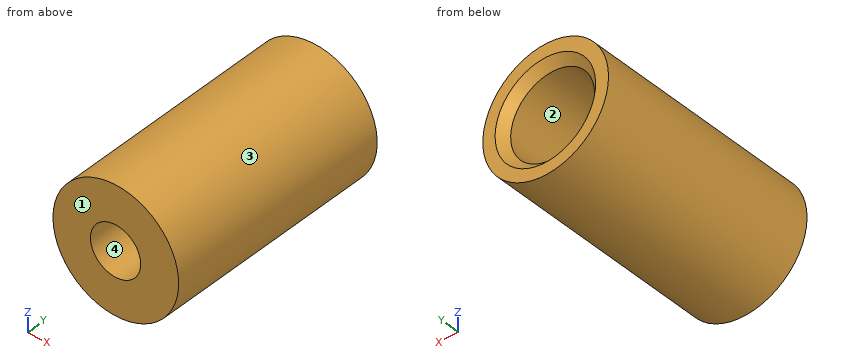
Autodesk Inventor part; units mm, degrees
ref_plane "YZ Plane" through (0, 0, 0) normal (1, 0, 0) x (0, 1, 0)
ref_plane "XZ Plane" through (0, 0, 0) normal (0, 1, 0) x (-1, 0, 0)
ref_plane "XY Plane" through (0, 0, 0) normal (0, 0, 1) x (1, 0, 0)
sketch "Эскиз1" plane through (0, 0, 0) normal (0, 1, 0) x (-1, 0, 0)
  circle A0 centre (0, 0) radius 15
  dimension "d0" = 30
extrude "Выдавливание1" add sketch "Эскиз1" along normal blind 55
hole "Отверстие1" at (-0.0551, 55, -0.1504) direction (0, -1, 0) diameter 12 depth 55 tip angle 118
hole "Отверстие2" at (0.0739, 55, -0.1164) direction (0, -1, 0) diameter 20 depth 25 tip angle 118
thread "Резьба1"
chamfer "Фаска1" distance 2 angle 45 1 edges at (0.0739, 55, -10.1164)
The listing builds one solid part. Answer for the finished solid, in the listing's coordinates (mm). Face numbers are marked on the shaded views. Round coordinates to 2 decimals unless told otherwise and drop trailing zeros. Write each loop counter-clockwise with the first axis right and the second up, starting at its lowest first coordinate (ties: lowest second). Pieces come first, ordered by that corner, then holes. Notation, with made-up numbers: M 47,35.5 L 55,35.5 A28 ccw 55,63.5 Z; hole C 4.25,46 d11. An arc over 180 degrees is marked long. Write each question's results on one line, items separated by ' | '. Start each with the question number.
Item 1: Find section B-B on y = 7.5. Write down the section's boundary in (x, z).
Item 2: Given pin 1 Ø14 at (x, z) = (-0.06, -0.15) entering from +Y; pin 2 Ø1.5 at (x, y) = (0.5, 49) entering from +Z; pin 3 Ø3 at (x, y) = (-10, 43) entering from +Z; pin 4 Ø2 at (y, z) = (25, -5) entering from -X, each flat-ended and moving along its own axis, determine where each tip first touches the part or whether it passes through.
Item 3: Find section A-A on x = -12.5. Write down the section's boundary in (y, z).
Item 4: Find section C-C on x = 13.25. Write down the section's boundary in (y, z).
Item 5: Straight lines are drawn through the part: probe 1 along X at (y, z) = (8.5, -4.75); probe 2 along X at (y, z) = (36, -8); probe 3 along Z at (x, y) = (-2, 22). For each, find the intervals that lie inside material, in ascending order.
Item 6: The mould has two halves that part along X. Classify the marked faces 1, 2, 3 and 4: +X half, -X half, draft (parallel to the pull), parting line (faces both ways), or undercut.
Answer block:
1) outline: C 0,0 d30; hole C -0.06,-0.15 d12
2) pin 1: stops at y = 28.28 | pin 2: stops at z = 15 | pin 3: stops at z = 12.36 | pin 4: stops at x = -14.46
3) outline: M 0,-8.29 L 55,-8.29 L 55,8.29 L 0,8.29 Z
4) outline: M 0,-7.03 L 55,-7.03 L 55,7.03 L 0,7.03 Z
5) probe 1: x = -14.23 to -3.91, 3.8 to 14.23 | probe 2: x = -12.69 to -6.08, 6.23 to 12.69 | probe 3: z = -14.87 to -5.83, 5.53 to 14.87
6) face 1: draft | face 2: undercut | face 3: parting line | face 4: undercut
